Design review of the part built by this model. Coordinates are the model's own, in mm. Face numbers are marked on the shaded views. A direction names the side the tool comes from. Round coordinates to 2 decimals unless told otherwise and drop trailing zeros. Order: outer loops, then holes, each group sorted by start corner. A loop starts at its lowest first (then second) coordinate and runs counter-clockwise, first axis right, second up. Notation, with made-up numbers: (-5, 89) - (1, 89) arc R11 ccw to (1, 93) - close; hole circle Ø2 at (69, 83). An arc over 180 degrees is marked (long way). Write item = value, one per line.
Autodesk Inventor part; units mm, degrees
ref_plane "YZ Plane" through (0, 0, 0) normal (1, 0, 0) x (0, 1, 0)
ref_plane "XZ Plane" through (0, 0, 0) normal (0, 1, 0) x (-1, 0, 0)
ref_plane "XY Plane" through (0, 0, 0) normal (0, 0, 1) x (1, 0, 0)
sketch "Sketch1" plane through (0, 0, 0) normal (0, 0, 1) x (1, 0, 0)
  line L0 (0, 9.6698) -> (0, -104.6302)
  line L1 (0, 9.6698) -> (76.2, 9.6698)
  line L2 (76.2, 9.6698) -> (76.2, -82.6078)
  arc A0 (0, -104.6302) -> (76.2, -82.6078) centre (11.8217, -2.6932) ccw
  point P0 (0, 0)
  dimension "d0" = 114.3
  dimension "d1" = 76.2
extrude "Extrusion1" add sketch "Sketch1" along normal blind 114.3
sketch "Sketch2" plane through (0, 9.6698, 0) normal (0, 1, 0) x (1, 0, 0)
  line L0 (72.2, -4) -> (4, -4)
  line L1 (4, -4) -> (4, -110.3)
  line L2 (4, -110.3) -> (72.2, -110.3)
  line L3 (72.2, -110.3) -> (72.2, -4)
  line L4 (76.2, -114.3) -> (0, -114.3)
  line L5 (76.2, 0) -> (0, 0)
  line L6 (76.2, 0) -> (76.2, -114.3)
  line L7 (0, 0) -> (0, -114.3)
  dimension "d4" = 4
  dimension "d5" = 4
  dimension "d6" = 4
  dimension "d7" = 4
extrude "Extrusion2" cut sketch "Sketch2" against normal blind 90 contours L3 L2 L1 L0
sketch "Sketch3" plane through (0, -104.6302, 0) normal (-1, 0, 0) x (0, 0, 1)
  circle A0 centre (19.05, 95.25) radius 2
  circle A1 centre (95.25, 95.25) radius 2
  circle A2 centre (19.05, 19.05) radius 2
  circle A3 centre (95.25, 19.05) radius 2
  line L0 (0, 114.3) -> (114.3, 114.3)
  line L1 (0, 114.3) -> (0, 0)
  line L2 (114.3, 114.3) -> (114.3, 0)
  line L3 (0, 0) -> (114.3, 0)
  point P0 (0, 104.6302)
  dimension "d10" = 4
  dimension "d11" = 4
  dimension "d12" = 4
  dimension "d13" = 4
  dimension "d14" = 19.05
  dimension "d15" = 19.05
  dimension "d16" = 19.05
  dimension "d17" = 19.05
  dimension "d18" = 19.05
  dimension "d19" = 19.05
  dimension "d20" = 19.05
  dimension "d21" = 19.05
extrude "Extrusion3" cut sketch "Sketch3" against normal blind 4 contours A0 | A1 | A2 | A3
equation "\"d22\" = d12"
properties part number "ashish1" material "PBT Plastic"
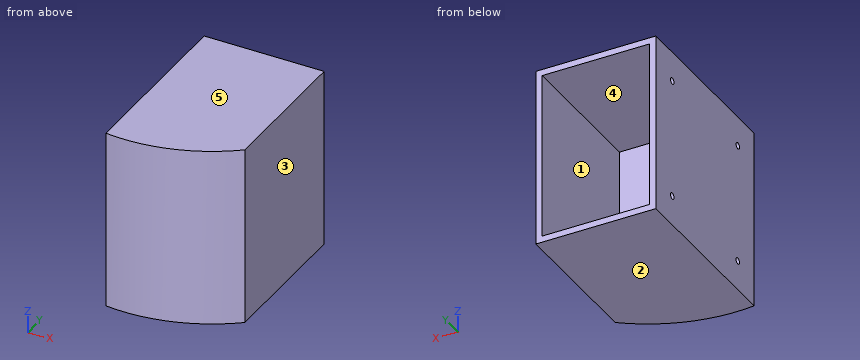
1) The part is to be moulded in two halves that separate along X. For the marked faces 3, 4 and 5, say which applies: released by +X, released by -X, zero draft, split by the parting line, or undercut.
Findings:
face_3 = released by +X
face_4 = undercut
face_5 = zero draft
2) To check wall thickness, follow L1, parallel to X at y = -62, z = 74.5; L2, parallel to Z at x = 58.5, y = -27.5; L3, parallel to Y at x = 2.5, z = 95.25. State the ranges of each line that lie inside material, in increasing order. Write a range as from..to.
Findings:
L1 = 0..4, 72.2..76.2
L2 = 0..4, 110.3..114.3
L3 = -104.89..-87.58, -83.58..-11.38, -7.38..9.67
3) We need section C-C on z = 104. Write out the cut boundary in (x, y).
Findings:
outline = (0, -104.63) arc R102.62 ccw to (76.2, -82.61) - (76.2, 9.67) - (72.2, 9.67) - (72.2, -80.33) - (4, -80.33) - (4, 9.67) - (0, 9.67) - close
4) We need section A-A on y = -69.5. Write out the cut boundary in (x, z).
Findings:
outline = (0, 0) - (76.2, 0) - (76.2, 114.3) - (0, 114.3) - close; hole (4, 4) - (72.2, 4) - (72.2, 110.3) - (4, 110.3) - close
5) We need section B-B on z = 19.05. Write out the cut boundary in (x, y).
Findings:
outline = (0, -104.63) arc R102.62 ccw to (76.2, -82.61) - (76.2, 9.67) - (72.2, 9.67) - (72.2, -80.33) - (4, -80.33) - (4, -11.38) - (0, -11.38) - (0, -83.58) - (4, -83.58) - (4, -87.58) - (0, -87.58) - close; (0, -7.38) - (4, -7.38) - (4, 9.67) - (0, 9.67) - close
6) For the marked faces 1 and 2, list the 3-axis set-ups (+Z, -Z, +X, -X, +Y, -Y) from which the entire face can be reached by the end or side of a thin tool; tool diameter is ignored.
Findings:
face_1 = +Y
face_2 = -Z, +X, -X, +Y, -Y
7) We need section D-D on x = 40.5. Write out the cut boundary in (y, z), and give its area (3 significant figures).
Findings:
outline = (-101.22, 0) - (9.67, 0) - (9.67, 4) - (-80.33, 4) - (-80.33, 110.3) - (9.67, 110.3) - (9.67, 114.3) - (-101.22, 114.3) - close
area = 3,110 mm^2
8) Clearance check with flat-ended pins moving along their axes: pin 1 Ø4.5 at (y, z) = (-85.58, 19.05) entering from +X; pin 2 Ø2 at (y, z) = (-85.5, 95.5) entering from -X; pin 3 Ø1.5 at (x, z) = (26.5, 50.5) entering from -Y. State where each tip first meets the part, or that it passes through.
Findings:
pin_1 = 75.29
pin_2 = 4
pin_3 = -104.36
